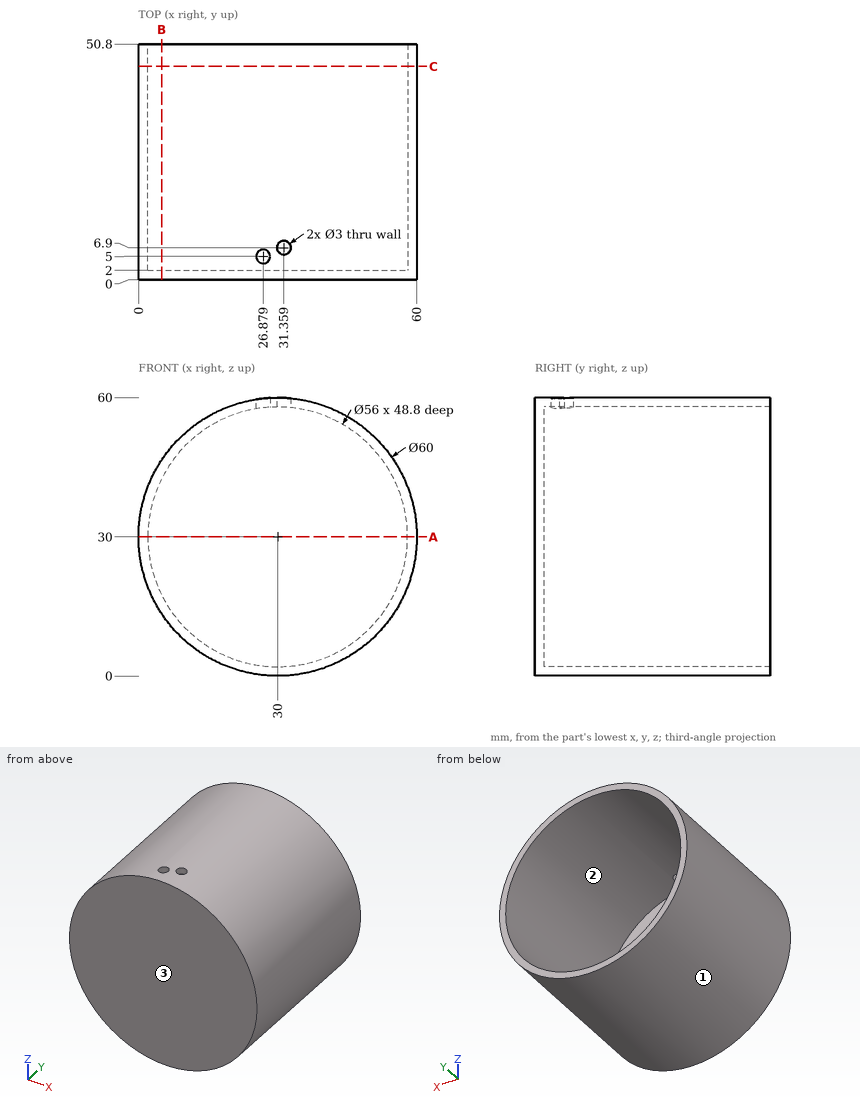
Input: dimensioned drawing with shaded views. Units: mm. Origin: part minimum x, y, z. Give positions to 0.01 mm unless a question says otherwise; leave off trailing zeros. Order: outer loops, then holes, each group sorted by start corner. A loop starts at its lowest first (then second) coordinate and runs counter-clockwise, first axis right, second up. Notation, with made-up numbers: (63.25, 73) -> (98.25, 73) arc R11 cw to (98.25, 86) -> close; hole circle Ø3 at (28.25, 28). An arc over 180 degrees is marked (long way). Use a Markdown table: item, result.
1) Ray query, line 1 along Z through (x, y) = (30.5, 13.5) (1 decimal); line 2 along Y through (x, z) = (34.5, 5.5); line 3 along X through (y, z) = (5, 52.5) (1 decimal). Return the intervals inside material, ascending. Write a range as [from, to].
Answer list:
| item | result |
|---|---|
| line 1 | [0, 2], [58, 60] |
| line 2 | [0, 2] |
| line 3 | [10.2, 13.3], [46.7, 49.8] |
2) Section query C-C, the plane y = 46. Return the cut outline in (x, z).
Answer list:
| item | result |
|---|---|
| outline | circle Ø60 at (30, 30); hole circle Ø56 at (30, 30) |
3) Section query A-A, the plane z = 30. Return the cut outline in (x, y), then the cut area to 3 significant figures.
Answer list:
| item | result |
|---|---|
| outline | (0, 0) -> (60, 0) -> (60, 50.8) -> (58, 50.8) -> (58, 2) -> (2, 2) -> (2, 50.8) -> (0, 50.8) -> close |
| area | 315 mm² |
4) Mould query, pull axis X, two halves, no side actions, for the marked faces 1, 2 and 3. Classes: +X half, -X half, draft (parallel to the pull), parting line (faces both ways), or undercut.
Answer list:
| item | result |
|---|---|
| face 1 | parting line |
| face 2 | undercut |
| face 3 | draft |
5) Section query B-B, the plane x = 5. Return the cut outline in (y, z), then the cut area to 3 significant figures.
Answer list:
| item | result |
|---|---|
| outline | (0, 13.42) -> (50.8, 13.42) -> (50.8, 17.39) -> (2, 17.39) -> (2, 42.61) -> (50.8, 42.61) -> (50.8, 46.58) -> (0, 46.58) -> close |
| area | 454 mm² |
6) Contact query for flat-ended pins moving along their axis: P1, Ø3, axis at y = 37.5, z = 8.5, coming from the +X side; P2, Ø4, axis at y = 23.5, z = 25.5, coming from the -X side; P3, Ø1.5, axis at x = 40, z = 12, coming from the +Y side. Output: stop coordinate, or through.
Answer list:
| item | result |
|---|---|
| P1 | x = 52.36 |
| P2 | x = 0.1 |
| P3 | y = 2 |
